Geometry: see drawing. Coordinates: mm, zero at the bounding-box minimum. A direction names the side the tool comes from. Coordinates: 2 decimals unless noted, no trailing zeros. Loops run counter-clockwise (first coordinate to the right, second up) from the corner with the lowest first, then second, coordinate; pieces in that order, holes last. Notation, with made-up numbers: (27.5, 17.25) -> (83.5, 17.25) arc R28 cw to (83.5, 42.25) -> close; hole circle Ø7 at (86, -19.5). An arc over 180 degrees is marked (long way). One line per item, written item: value. Start each with the question number.
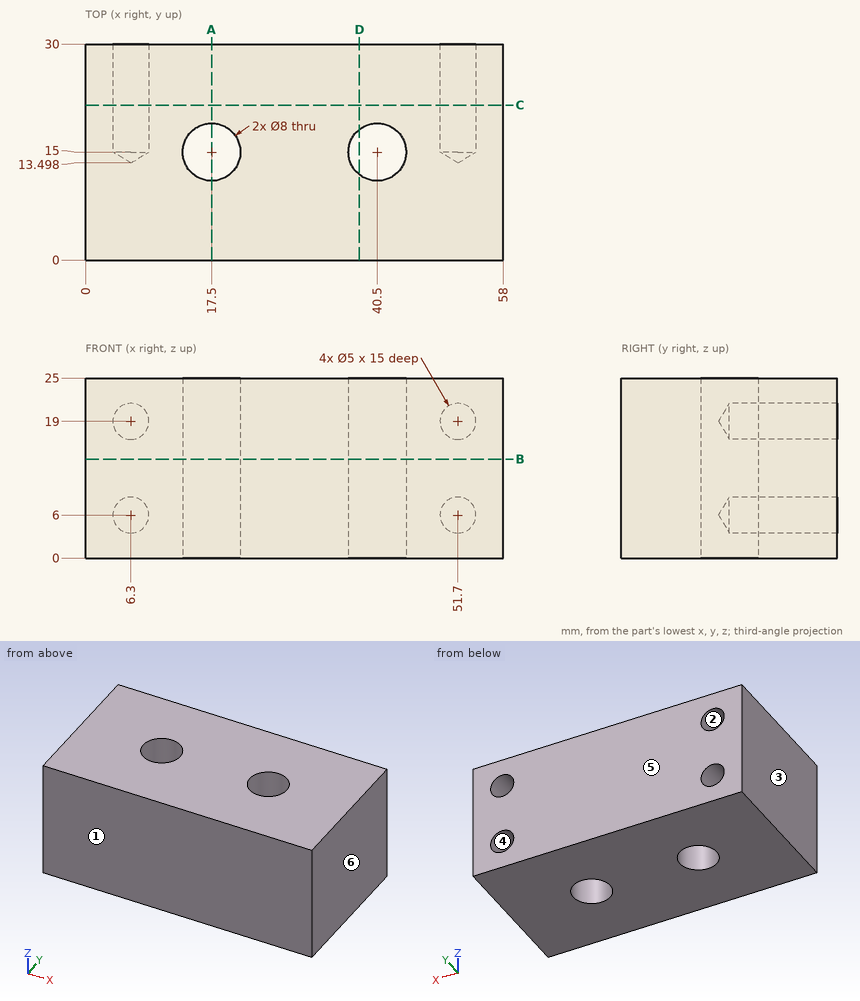
1. Section B-B on z = 13.75. Return the cut outline in (x, y).
2. Section C-C on y = 21.5. Return the cut outline in (x, z), plus the area to 3 significant figures.
3. Section A-A on x = 17.5. Return the cut outline in (y, z).
4. Section D-D on x = 38. Return the cut outline in (y, z).
5. Line query: L1, parallel to X at y = 19.75, z = 19; L2, parallel to Z at x = 6.3, y = 19.75; L3, parallel to Y at x = 17.5, z = 11.5. Output: solid intervals per line, ascending. Write a range as [from, to].
6. Set-up query: the marked faces 1 and 2. Return all of +Z, -Z, +X, -X, +Y, -Y with unobstructed straight access to the full face (end or side cutting, diameter ignored); none if empty.
7. Pin query (flat end, axial travel): pin 1 Ø4 at (x, y) = (22, 21.5) entering from -Z; pin 2 Ø3 at (x, z) = (51.7, 6) entering from +Y; pin 3 Ø4 at (x, z) = (6.3, 19) entering from +Y. Return the tip coordinate at first contact, or that it passes through.
8. Draft query along X for the marked faces 3, 4, 5 and 6. Return one class per face: released by +X, released by -X, zero draft, split by the parting line, or undercut.
Checks:
1. outline: (0, 0) -> (58, 0) -> (58, 30) -> (0, 30) -> close; hole circle Ø8 at (17.5, 15); hole circle Ø8 at (40.5, 15)
2. outline: (0, 0) -> (58, 0) -> (58, 25) -> (0, 25) -> close; hole circle Ø5 at (6.3, 6); hole circle Ø5 at (6.3, 19); hole circle Ø5 at (51.7, 6); hole circle Ø5 at (51.7, 19)
2. area: 1,370 mm²
3. outline: (0, 0) -> (11, 0) -> (11, 25) -> (0, 25) -> close; (19, 0) -> (30, 0) -> (30, 25) -> (19, 25) -> close
4. outline: (0, 0) -> (11.88, 0) -> (11.88, 25) -> (0, 25) -> close; (18.12, 0) -> (30, 0) -> (30, 25) -> (18.12, 25) -> close
5. L1: [0, 3.8], [8.8, 49.2], [54.2, 58]
5. L2: [0, 3.5], [8.5, 16.5], [21.5, 25]
5. L3: [0, 11], [19, 30]
6. face 1: +Z, -Z, +X, -X, -Y
6. face 2: +Y
7. pin 1: z = 0
7. pin 2: y = 14.4
7. pin 3: y = 14.7
8. face 3: released by -X
8. face 4: undercut
8. face 5: zero draft
8. face 6: released by +X
